Build history of the part. All positions in model axes, mm. A direction names the side the tool comes from. Give positions to 0.01 mm unless a question says otherwise; leave off trailing zeros. Order: outer loops, then holes, each group sorted by start corner. A loop starts at its lowest first (then second) coordinate and runs counter-clockwise, first axis right, second up. Notation, with made-up numbers: (67, 40) - (126, 40) arc R21 cw to (126, 76) - close; hole circle Ø1 at (89, 45). An arc over 180 degrees is marked (long way). Use a Markdown table: item, result.
Autodesk Inventor part; units mm, degrees
ref_plane "YZ Plane" through (0, 0, 0) normal (1, 0, 0) x (0, 1, 0)
ref_plane "XZ Plane" through (0, 0, 0) normal (0, 1, 0) x (-1, 0, 0)
ref_plane "XY Plane" through (0, 0, 0) normal (0, 0, 1) x (1, 0, 0)
sketch "Sketch1" plane through (0, 0, 0) normal (0, 1, 0) x (-1, 0, 0)
  line L0 (0, 0) -> (26.5, 0)
  line L1 (26.5, 0) -> (26.5, -33)
  line L2 (26.5, -33) -> (0, -33)
  line L3 (0, -33) -> (0, 0)
  line L4 (26.5, -33) -> (26.5, -30)
  line L5 (26.5, -30) -> (0, -30)
  circle A0 centre (13.25, -13.25) radius 4
  arc A1 (22.5449, -12.2666) -> (20.6583, -12.6119) centre (21.75, -13.25) ccw
  circle A2 centre (21.75, -13.25) radius 1.6
  circle A3 centre (4.75, -13.25) radius 1.75
  circle A4 centre (4.75, -13.25) radius 1.6
  circle A5 centre (13.25, -13.25) radius 13.25
  line L6 (13.25, -13.25) -> (13.25, 0)
  line L7 (13.25, 0) -> (13.25, -13.25)
  point P0 (0, -13.25)
  point P1 (26.5, -13.25)
  dimension "d9" = 26.5
  dimension "d3" = 26.5
  dimension "d4" = 33
  dimension "d5" = 3
  dimension "d6" = 8
  dimension "d7" = 3.2
  dimension "d8" = 3.2
  dimension "d10" = 13.25
extrude "Extrusion1" add sketch "Sketch1" along normal blind 3 contours A5 | A5 L1 L5 L3 | L5 L1 L2 L3
sketch "Sketch2" plane through (0, 0, 0) normal (0, -1, 0) x (1, 0, 0)
  line L0 (0, -33) -> (-26.5, -33)
  line L1 (0, -13.25) -> (0, -33)
  line L2 (-26.5, -33) -> (0, -33)
  line L3 (0, -33) -> (0, -30)
  line L4 (0, -30) -> (-26.5, -30)
  line L5 (-26.5, -30) -> (-26.5, -33)
  point P0 (0, 0)
  dimension "d13" = 3
extrude "Extrusion2" add sketch "Sketch2" along normal blind 33
fillet "Fillet1" radius 2 1 edges at (-13.25, 3, -33)
sketch "Sketch3" plane through (-26.5, 0, -30) normal (0, 0, 1) x (1, 0, 0)
  line L0 (26.5, -33) -> (0, -33)
  line L1 (13.25, -33) -> (13.25, 0)
  line L2 (0, 0) -> (0, -33)
  line L3 (0, -16.5) -> (26.5, -16.5)
  line L4 (26.5, 0) -> (26.5, -33)
  circle A0 centre (13.25, -16.5) radius 5
  line L5 (0, -16.5) -> (0, -23.5)
  line L6 (13.25, -33) -> (5.25, -33)
  circle A1 centre (5.25, -23.5) radius 1.8
  circle A2 centre (5.25, -9.5) radius 1.8
  circle A3 centre (21.25, -23.5) radius 1.8
  circle A4 centre (21.25, -9.5) radius 1.8
  dimension "d17" = 10
  dimension "d18" = 7
  dimension "d19" = 8
  dimension "d20" = 3.6
  dimension "d23" = 14
  dimension "d26" = 16
extrude "Extrusion3" cut sketch "Sketch3" against normal blind 33 contours A0 L3 L1 | L1 L3 A0 | L3 L1 A0 | L3 A0 L1 | A1 | A2 | A3 | A4
sketch "Sketch4" plane through (-26.5, 0, -30) normal (0, 0, 1) x (1, 0, 0)
  line L0 (0, -33) -> (0, 1)
  line L1 (26.5, 0) -> (0, 0)
  line L2 (0, 0) -> (0, -33)
  line L3 (0, -33) -> (26.5, -33)
  line L4 (26.5, -33) -> (26.5, 0)
  circle A0 centre (13.25, -16.5) radius 5
  circle A1 centre (21.25, -23.5) radius 1.8
  circle A2 centre (21.25, -23.5) radius 1.8
  circle A3 centre (21.25, -9.5) radius 1.8
  circle A4 centre (21.25, -9.5) radius 1.8
  circle A5 centre (5.25, -9.5) radius 1.8
  circle A6 centre (5.25, -9.5) radius 1.8
  circle A7 centre (5.25, -23.5) radius 1.8
  circle A8 centre (5.25, -23.5) radius 1.8
  line L5 (26.5, 0) -> (0, 0)
  line L6 (0, 0) -> (0, -33)
  line L7 (0, -33) -> (26.5, -33)
  line L8 (26.5, -33) -> (26.5, 0)
sketch "Sketch5" plane through (-26.5, 0, -30) normal (0, 0, 1) x (1, 0, 0)
  line L0 (0, -33) -> (0, 1)
  line L1 (26.5, -33) -> (26.5, 1)
  line L2 (0, 0) -> (26.5, 0)
  line L3 (26.5, 0) -> (26.5, -3)
  line L4 (26.5, -3) -> (0, -3)
  line L5 (0, -3) -> (0, 0)
  dimension "d31" = 3
extrude "Extrusion4" add sketch "Sketch5" along normal blind 30
sketch "Sketch6" plane through (-13.25, 0, -13.25) normal (0, 1, 0) x (1, 0, 0)
  circle A0 centre (0, 0) radius 4
  circle A1 centre (-8.5, 0) radius 1.6
  circle A2 centre (-8.5, 0) radius 1.6
  circle A3 centre (8.5, 0) radius 1.75
  circle A4 centre (8.5, 0) radius 1.75
  point P0 (13.25, -13.25)
properties part number "bracket jga"
1) Two-plate mould, pull along Z, no slides. Class faces 1 (the cylindrical face through (-13.06, 2.4, -32.43)), 2 (the flat face through (-13, 0, -13)), 3 (the flat face through (-13, -3, -15)): +Z half, -Z half, draft (parallel to the pull), parting line (faces both ways), or undercut.
Computed:
| item | result |
|---|---|
| face 1 | -Z half |
| face 2 | undercut |
| face 3 | draft |
2) Tool access for faces 4 (the flat face through (-10, -12, -33)), 5 (the flat face through (-24, 0, -3)), 6 (the flat face through (-10, -21, -30)), 7 (the flat face through (-3, 0, -3)), 8 (the cylindrical face through (-4.522, 1.479, -14.985)): list every direction of +Z, -Z, +X, -X, +Y, -Y with a clear straight run to the whole face (end or side of a thin tool).
Computed:
| item | result |
|---|---|
| face 4 | -Z, +X, -X, +Y, -Y |
| face 5 | +Z, -X, +Y |
| face 6 | +Z, +X, -X, -Y |
| face 7 | +Z, +X, +Y |
| face 8 | +Y |
3) Slice it at C-C (y = -16.5). Write the cut outline in (x, z), and give its area (3 significant figures).
Computed:
| item | result |
|---|---|
| outline | (-26.5, -33) - (-18.25, -33) - (-18.25, -30) - (-26.5, -30) - close; (-8.25, -33) - (0, -33) - (0, -30) - (-8.25, -30) - close |
| area | 49.5 mm² |
4) Slice it at A-A (y = -23.5). Write the cut outline in (x, z).
Computed:
| item | result |
|---|---|
| outline | (-26.5, -33) - (-23.05, -33) - (-23.05, -30) - (-26.5, -30) - close; (-19.45, -33) - (-7.05, -33) - (-7.05, -30) - (-19.45, -30) - close; (-3.45, -33) - (0, -33) - (0, -30) - (-3.45, -30) - close |
5) Slice it at B-B (x = -21.75). Write the cut outline in (y, z), and give its area (3 significant figures).
Computed:
| item | result |
|---|---|
| outline | (-33, -33) - (-25.23, -33) - (-25.23, -30) - (-33, -30) - close; (-21.77, -33) - (-11.23, -33) - (-11.23, -30) - (-21.77, -30) - close; (-7.77, -33) - (1, -33) arc R2 ccw to (3, -31) - (3, -14.85) - (0, -14.85) - (0, -11.65) - (3, -11.65) - (3, -3.09) - (0, -3.09) - (0, 0) - (-3, 0) - (-3, -30) - (-7.77, -30) - close |
| area | 248 mm² |
6) Wall check: line 1 (Y direction, x = -21.25, z = -30.85); line 2 (Y direction, x = -21.25, z = -31.5); line 3 (Y direction, x = -6.75, z = -11.5). Give the ranges that are in metal, low to high. Write a range as from..to.
Computed:
| item | result |
|---|---|
| line 1 | y = -33..-25.3, -21.7..-11.3, -7.7..3 |
| line 2 | y = -33..-25.3, -21.7..-11.3, -7.7..2.94 |
| line 3 | y = -3..3 |
7) Pin check, flat tips, straight feed: P1, Ø3, axis at x = -5.25, y = -23.5, coming from the -Z side; P2, Ø5, axis at x = -21, z = -6.5, coming from the -Y side; P3, Ø1, axis at x = -22.5, z = -13.5, coming from the +Y side; P4, Ø13, axis at x = -12.5, y = -14, coming from the +Z side. Stop position of each tip, or through.
Computed:
| item | result |
|---|---|
| P1 | passes through |
| P2 | stops at y = -3 |
| P3 | stops at y = 0 |
| P4 | stops at z = -30 |
8) Slice it at D-D (z = -2). Write the cut outline in (x, y), and give its area (4 significant figures).
Computed:
| item | result |
|---|---|
| outline | (-26.5, -3) - (0, -3) - (0, 0) - (-6.25, 0) - (-6.25, 3) - (-20.25, 3) - (-20.25, 0) - (-26.5, 0) - close |
| area | 121.5 mm² |
